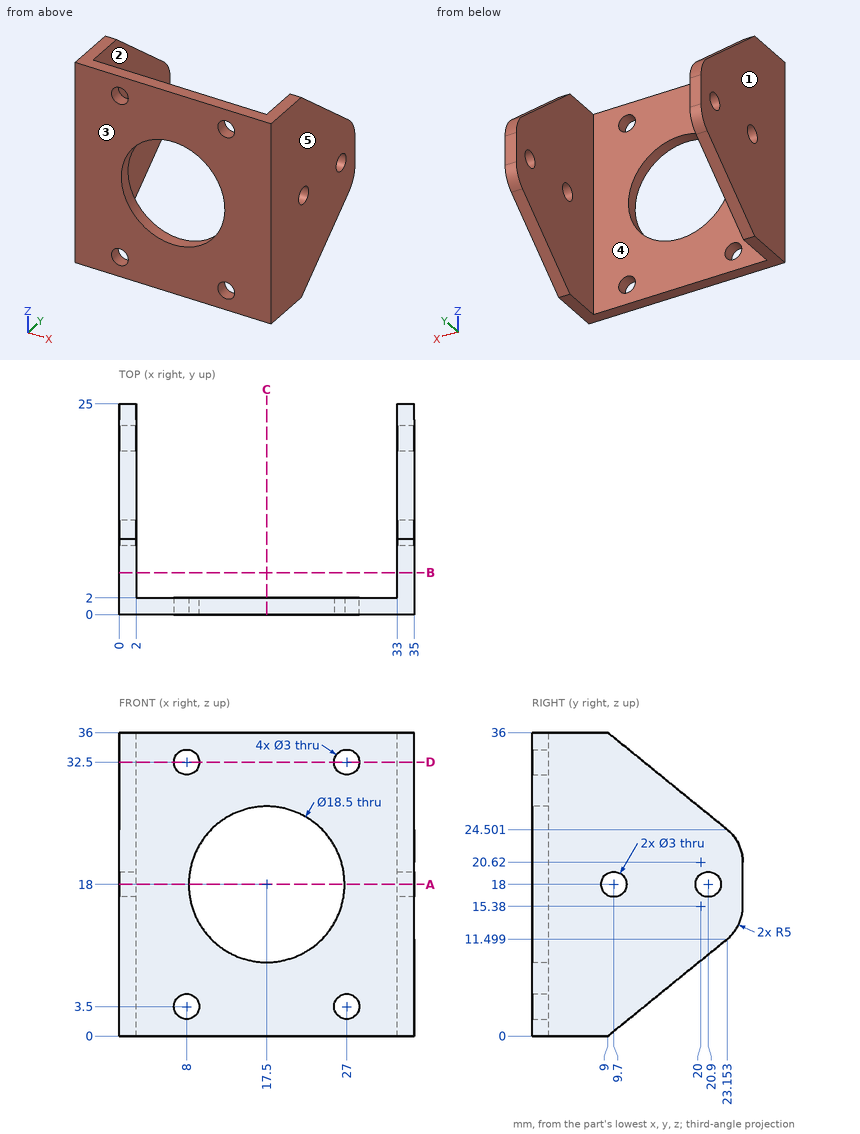
Geometry check sheet. Reference: drawing and pictorial views, mm from the part's lowest x, y, z. A direction names the side the tool comes from. Coordinates: 2 decimals unless noted, no trailing zeros. Order: outer loops, then holes, each group sorted by start corner. A loop starts at its lowest first (then second) coordinate and runs counter-clockwise, first axis right, second up. Notation, with made-up numbers: M 89,0 L 147,0 A16 cw 147,31 Z; hole C 86,16.25 d8. An arc over 180 degrees is marked long. Return JSON: item names as keys, results as strings.
1) Cross-section at C-C, the plane x = 17.5. Record the boundary of the cut face in (y, z).
Answer list:
{"outline": "M 0,0 L 2,0 L 2,8.75 L 0,8.75 Z; M 0,27.25 L 2,27.25 L 2,36 L 0,36 Z"}
2) Cross-section at D-D, the plane z = 32.5. Record the boundary of the cut face in (x, y), and give its area (3 significant figures).
Answer list:
{"outline": "M 0,0 L 6.5,0 L 6.5,2 L 2,2 L 2,13.31 L 0,13.31 Z; M 9.5,0 L 25.5,0 L 25.5,2 L 9.5,2 Z; M 28.5,0 L 35,0 L 35,13.31 L 33,13.31 L 33,2 L 28.5,2 Z", "area": "103 mm2"}
3) Gauge pin test, flat ends, axial feed: pin 1 (1 mm diameter, centred on x = 31, z = 17.5, fed in from -Y); pin 2 (4 mm diameter, centred on x = 27, z = 32.5, fed in from +Y); pin 3 (2 mm diameter, centred on x = 17.5, y = 4.5, fed in from -Z). Record the tip position at first contact, or that the pin passes through.
Answer list:
{"pin 1": "y = 0", "pin 2": "y = 2", "pin 3": "through"}
4) Cross-section at B-B, the plane y = 5. Record the boundary of the cut face in (x, z), and give its area (3 significant figures).
Answer list:
{"outline": "M 0,0 L 2,0 L 2,36 L 0,36 Z; M 33,0 L 35,0 L 35,36 L 33,36 Z", "area": "144 mm2"}
5) Cross-section at A-A, the plane z = 18. Record the boundary of the cut face in (x, y).
Answer list:
{"outline": "M 0,0 L 8.25,0 L 8.25,2 L 2,2 L 2,8.2 L 0,8.2 Z; M 0,11.2 L 2,11.2 L 2,19.4 L 0,19.4 Z; M 0,22.4 L 2,22.4 L 2,25 L 0,25 Z; M 26.75,0 L 35,0 L 35,8.2 L 33,8.2 L 33,2 L 26.75,2 Z; M 33,11.2 L 35,11.2 L 35,19.4 L 33,19.4 Z; M 33,22.4 L 35,22.4 L 35,25 L 33,25 Z"}
6) Thickness scan on L1, parallel to Y at x = 33.55, z = 18; L2, parallel to Z at x = 27, y = 1.6; L3, parallel to X at y = 14.5, z = 7. Record the ranges inside material, lowest first. Write a range as [from, to].
Answer list:
{"L1": "[0, 8.2], [11.2, 19.4], [22.4, 25]", "L2": "[0, 2], [5, 31], [34, 36]", "L3": "[0, 2], [33, 35]"}
7) Access from +Z, -Z, +X, -X, +Y, -Y to the whole of each face (thin tool, end or side, straight path). Record for the marked faces 4 and 5.
Answer list:
{"face 4": "+Z, -Z, +Y", "face 5": "+Z, -Z, +X, +Y, -Y"}
8) Release check for a two-part mould opening along X. For the marked faces 1, 2 and 3 record: +X half, -X half, draft (parallel to the pull), parting line (faces both ways), or undercut.
Answer list:
{"face 1": "-X half", "face 2": "undercut", "face 3": "draft"}
